Model file for the job. Use its own axes, mm. Face numbers are marked on the shaded views. A direction names the side the tool comes from. Round coordinates to 2 decimals unless told otherwise and drop trailing zeros. Loops run counter-clockwise (first coordinate to the right, second up) from the corner with the lowest first, then second, coordinate; pieces in that order, holes last. Notation, with made-up numbers: (46, -7) -> (84, -7) arc R20 cw to (84, 0) -> close; hole circle Ø2 at (54, 17). An arc over 180 degrees is marked (long way). Use a Markdown table: item, result. Add a question column.
```python
from build123d import *

# Parameters (mm, degrees)
BASE_SKETCH_W       = 60
BASE_SKETCH_H       = 60
BASE_SKETCH_R       = 12.5
BOSS_EXTRUDE1_DEPTH = 10
BASE_SKETCH_3_R     = 12.5
BOSS_EXTRUDE2_DEPTH = 20


with BuildPart() as part:
    # Base Sketch → Boss-Extrude1 (new body)
    # profile 1 of 2: a face of its own
    with BuildSketch(Plane.XY):
        Polygon((-70, -15), (-55, -30), (-30, -30), (-30, 30), (-55, 30), (-70, 15), align=None)
    # profile 2 of 2: a face of its own
    with BuildSketch(Plane.XY):
        Rectangle(BASE_SKETCH_W, BASE_SKETCH_H)
        Circle(BASE_SKETCH_R, mode=Mode.SUBTRACT)
    extrude(amount=BOSS_EXTRUDE1_DEPTH)

    # Base Sketch_3 → Boss-Extrude2 (add)
    with BuildSketch(Plane.XY):
        Circle(BASE_SKETCH_3_R)
    extrude(amount=BOSS_EXTRUDE2_DEPTH)


solid = part.part
```
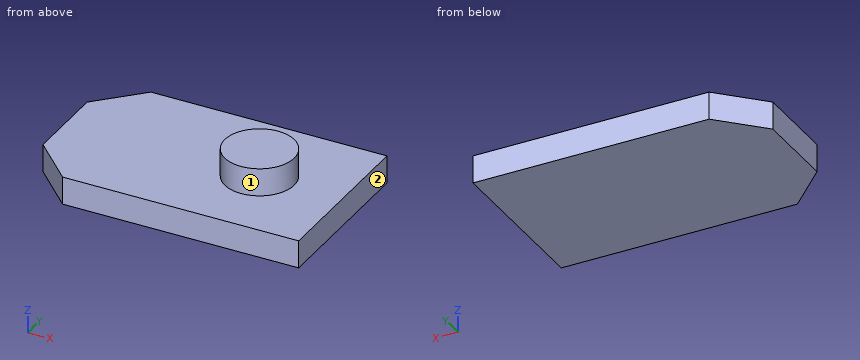
1) Tool access for the marked faces 1 and 2: list every direction of +Z, -Z, +X, -X, +Y, -Y with a clear straight run to the whole face (end or side of a thin tool).
2) Wall check: probe 1 along Z at (x, y) = (-26, 6); probe 2 along X at (y, z) = (-11, 13.5); probe 3 along X at (y, z) = (-24.5, 4.5). Give the ranges that are in metal, low to high. Write a range as from..to.
3) Cut at C-C on z = 13. Write the cut outline in (x, y).
4) Pin check, flat tips, straight feed: pin 1 Ø3 at (y, z) = (-10, 16) entering from +X; pin 2 Ø1 at (y, z) = (-1.5, 11) entering from -X. Stop position of each tip, or through.
5) Cut at A-A on y = 0. Write the cut outline in (x, z).
6) Cut at D-D on y = 25.5. Write the cut outline in (x, z).
7) Cut at B-B on x = 0. Write the cut outline in (y, z), and give its area (3 significant figures).
Established:
| question | item | result |
|---|---|---|
| 1 | face 1 | +Z |
| 1 | face 2 | +Z, -Z, +X, +Y, -Y |
| 2 | probe 1 | z = 0..10 |
| 2 | probe 2 | x = -5.94..5.94 |
| 2 | probe 3 | x = -60.5..30 |
| 3 | outline | circle Ø25 at (0, 0) |
| 4 | pin 1 | stops at x = 9.17 |
| 4 | pin 2 | stops at x = -12.46 |
| 5 | outline | (-70, 0) -> (30, 0) -> (30, 10) -> (12.5, 10) -> (12.5, 20) -> (-12.5, 20) -> (-12.5, 10) -> (-70, 10) -> close |
| 6 | outline | (-59.5, 0) -> (30, 0) -> (30, 10) -> (-59.5, 10) -> close |
| 7 | outline | (-30, 0) -> (30, 0) -> (30, 10) -> (12.5, 10) -> (12.5, 20) -> (-12.5, 20) -> (-12.5, 10) -> (-30, 10) -> close |
| 7 | area | 850 mm^2 |
